Read the model definition and answer for the solid it produces. Units are mm, in the model's axes. Face numbers are marked on the shaded views. A direction names the side the tool comes from. Round coordinates to 2 decimals unless told otherwise and drop trailing zeros. Write each loop counter-clockwise with the first axis right and the second up, starting at its lowest first coordinate (ties: lowest second). Pieces come first, ordered by that corner, then holes. Notation, with made-up numbers: (-1.75, 47.25) -> (9.25, 47.25) arc R18 cw to (9.25, 72.25) -> close; hole circle Ø3 at (55, 40.5). An arc over 180 degrees is marked (long way). Return JSON: item names as keys, results as strings.
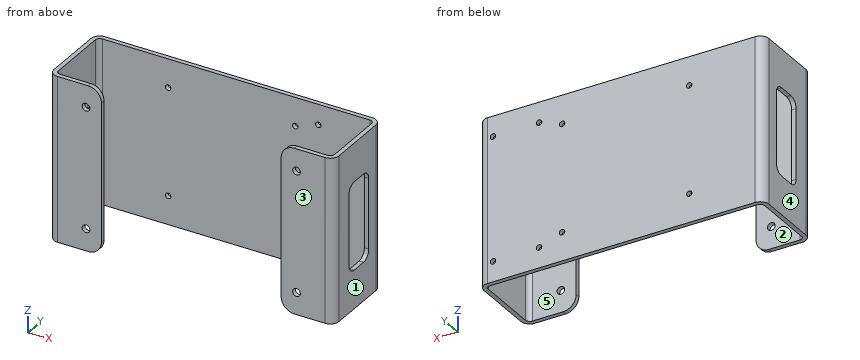
from build123d import *

# Parameters (mm, degrees)
SKETCH1_W                    = 130
SKETCH1_H                    = 75
BASE_FLANGE1_DEPTH           = 2
EDGE_FLANGE1_STRIP_W         = 12
EDGE_FLANGE1_STRIP_H         = 2
EDGE_FLANGE1_STRIP_CUT_DEPTH = 75
EDGE_FLANGE1_DEPTH           = 75
EDGE_FLANGE2_STRIP_W         = 12
EDGE_FLANGE2_STRIP_H         = 2
EDGE_FLANGE2_STRIP_CUT_DEPTH = 75
EDGE_FLANGE2_DEPTH           = 75
EDGE_FLANGE3_STRIP_W         = 12
EDGE_FLANGE3_STRIP_H         = 2
EDGE_FLANGE3_STRIP_CUT_DEPTH = 75
EDGE_FLANGE3_DEPTH           = 75
EDGE_FLANGE4_STRIP_W         = 12
EDGE_FLANGE4_STRIP_H         = 2
EDGE_FLANGE4_STRIP_CUT_DEPTH = 75
EDGE_FLANGE4_DEPTH           = 75
SKETCH20_R                   = 1.75
CUT_EXTRUDE1_DEPTH           = 2
CUT_EXTRUDE2_DEPTH           = 128
FILLET1_R                    = 6
SKETCH22_R                   = 1.25
CUT_EXTRUDE3_DEPTH           = 2
SKETCH23_R                   = 1.25
CUT_EXTRUDE4_DEPTH           = 2


# Sheet-metal steps are written as plain solids
with BuildPart() as part:
    # Sketch1 → Base-Flange1 (new body)
    with BuildSketch(Plane(origin=(0, 0, 0), x_dir=(1, 0, 0), z_dir=(0, 1, 0))):
        Rectangle(SKETCH1_W, SKETCH1_H)
    extrude(amount=-BASE_FLANGE1_DEPTH)

    # Edge-Flange1 strip (across the edge) → Edge-Flange1 strip cut (cut)
    with BuildSketch(Plane(origin=(-65, -2, 37.5), x_dir=(1, 0, 0), z_dir=(0, 0, -1))):
        with Locations((-2, -1)):
            Rectangle(EDGE_FLANGE1_STRIP_W, EDGE_FLANGE1_STRIP_H)
    extrude(amount=EDGE_FLANGE1_STRIP_CUT_DEPTH, mode=Mode.SUBTRACT)

    # Edge-Flange1 section (across the edge) → Edge-Flange1 (add)
    with BuildSketch(Plane(origin=(-65, -2, 37.5), x_dir=(1, 0, 0), z_dir=(0, 0, -1))):
        with BuildLine():
            Line((0, 2), (0, 32))
            Line((0, 32), (2, 32))
            Line((2, 32), (2, 2))
            ThreePointArc((2, 2), (2.585786438, 0.585786438), (4, 0))
            Line((4, 0), (4, -2))
            ThreePointArc((4, -2), (1.171572875, -0.828427125), (0, 2))
        make_face()
    extrude(amount=EDGE_FLANGE1_DEPTH)

    # Edge-Flange2 strip (across the edge) → Edge-Flange2 strip cut (cut)
    with BuildSketch(Plane(origin=(-63, -34, 37.5), x_dir=(0, 1, 0), z_dir=(0, 0, -1))):
        with Locations((-4, -1)):
            Rectangle(EDGE_FLANGE2_STRIP_W, EDGE_FLANGE2_STRIP_H)
    extrude(amount=EDGE_FLANGE2_STRIP_CUT_DEPTH, mode=Mode.SUBTRACT)

    # Edge-Flange2 section (across the edge) → Edge-Flange2 (add)
    with BuildSketch(Plane(origin=(-63, -34, 37.5), x_dir=(0, 1, 0), z_dir=(0, 0, -1))):
        with BuildLine():
            Line((-2, 2), (-2, 22))
            Line((-2, 22), (0, 22))
            Line((0, 22), (0, 2))
            ThreePointArc((0, 2), (0.585786438, 0.585786438), (2, 0))
            Line((2, 0), (2, -2))
            ThreePointArc((2, -2), (-0.828427125, -0.828427125), (-2, 2))
        make_face()
    extrude(amount=EDGE_FLANGE2_DEPTH)

    # Edge-Flange3 strip (across the edge) → Edge-Flange3 strip cut (cut)
    with BuildSketch(Plane(origin=(65, -2, -37.5), x_dir=(-1, 0, 0), z_dir=(0, 0, 1))):
        with Locations((-2, -1)):
            Rectangle(EDGE_FLANGE3_STRIP_W, EDGE_FLANGE3_STRIP_H)
    extrude(amount=EDGE_FLANGE3_STRIP_CUT_DEPTH, mode=Mode.SUBTRACT)

    # Edge-Flange3 section (across the edge) → Edge-Flange3 (add)
    with BuildSketch(Plane(origin=(65, -2, -37.5), x_dir=(-1, 0, 0), z_dir=(0, 0, 1))):
        with BuildLine():
            Line((0, 2), (0, 32))
            Line((0, 32), (2, 32))
            Line((2, 32), (2, 2))
            ThreePointArc((2, 2), (2.585786438, 0.585786438), (4, 0))
            Line((4, 0), (4, -2))
            ThreePointArc((4, -2), (1.171572875, -0.828427125), (0, 2))
        make_face()
    extrude(amount=EDGE_FLANGE3_DEPTH)

    # Edge-Flange4 strip (across the edge) → Edge-Flange4 strip cut (cut)
    with BuildSketch(Plane(origin=(63, -34, -37.5), x_dir=(0, 1, 0), z_dir=(0, 0, 1))):
        with Locations((-4, -1)):
            Rectangle(EDGE_FLANGE4_STRIP_W, EDGE_FLANGE4_STRIP_H)
    extrude(amount=EDGE_FLANGE4_STRIP_CUT_DEPTH, mode=Mode.SUBTRACT)

    # Edge-Flange4 section (across the edge) → Edge-Flange4 (add)
    with BuildSketch(Plane(origin=(63, -34, -37.5), x_dir=(0, 1, 0), z_dir=(0, 0, 1))):
        with BuildLine():
            Line((-2, 2), (-2, 22))
            Line((-2, 22), (0, 22))
            Line((0, 22), (0, 2))
            ThreePointArc((0, 2), (0.585786438, 0.585786438), (2, 0))
            Line((2, 0), (2, -2))
            ThreePointArc((2, -2), (-0.828427125, -0.828427125), (-2, 2))
        make_face()
    extrude(amount=EDGE_FLANGE4_DEPTH)

    # Sketch20 → Cut-Extrude1 (cut)
    with BuildSketch(Plane(origin=(0, -34, 0), x_dir=(1, 0, 0), z_dir=(0, 1, 0))):
        with Locations(Location((-48, -27.5, 0), (0, 0, 180))):
            Circle(SKETCH20_R)
        with Locations(Location((-48, 27.5, 0), (0, 0, 180))):
            Circle(SKETCH20_R)
    cut_extrude1 = extrude(amount=-CUT_EXTRUDE1_DEPTH, mode=Mode.SUBTRACT)

    # Sketch21 → Cut-Extrude2 (cut)
    with BuildSketch(Plane.ZY.offset(65)):
        with BuildLine():
            Line((-16, -9.5), (16, -9.5))
            ThreePointArc((16, -9.5), (18.828427125, -10.671572875), (20, -13.5))
            Line((20, -13.5), (20, -20.5))
            ThreePointArc((20, -20.5), (18.828427125, -23.328427125), (16, -24.5))
            Line((16, -24.5), (-16, -24.5))
            ThreePointArc((-16, -24.5), (-18.828427125, -23.328427125), (-20, -20.5))
            Line((-20, -20.5), (-20, -13.5))
            ThreePointArc((-20, -13.5), (-18.828427125, -10.671572875), (-16, -9.5))
        make_face()
    cut_extrude2 = extrude(amount=-CUT_EXTRUDE2_DEPTH, mode=Mode.SUBTRACT)

    # Fillet1
    fillet1_edges = [part.edges().sort_by_distance(p)[0] for p in [
        (41, -35, -37.5),
        (41, -35, 37.5),
        (-41, -35, 37.5),
        (-41, -35, -37.5),
    ]]
    fillet(fillet1_edges, radius=FILLET1_R)

    # Mirror4: Cut-Extrude1, Cut-Extrude2 across plane
    add(cut_extrude1.mirror(Plane(origin=(0, 0, 0), x_dir=(0, 0, 1), z_dir=(1, 0, 0))), mode=Mode.SUBTRACT)
    add(cut_extrude2.mirror(Plane(origin=(0, 0, 0), x_dir=(0, 0, 1), z_dir=(1, 0, 0))), mode=Mode.SUBTRACT)

    # Sketch22 → Cut-Extrude3 (cut)
    with BuildSketch(Plane(origin=(0, 0, 0), x_dir=(1, 0, 0), z_dir=(0, 1, 0))):
        with BuildLine():
            Line((-31, 23.25), (-31, 24.5))
            Line((-31, 24.5), (-29.75, 24.5))
            ThreePointArc((-29.75, 24.5), (-31.883883476, 25.383883476), (-31, 23.25))
        make_face()
        with BuildLine():
            Line((-29.75, 24.5), (-31, 24.5))
            Line((-31, 24.5), (-31, 23.25))
            ThreePointArc((-31, 23.25), (-30.116116524, 23.616116524), (-29.75, 24.5))
        make_face()
        with Locations(Location((27, 24.5, 0), (0, 0, 270))):
            Circle(SKETCH22_R)
        with Locations(Location((27, -24.5, 0), (0, 0, 270))):
            Circle(SKETCH22_R)
        with Locations(Location((-31, -24.5, 0), (0, 0, 270))):
            Circle(SKETCH22_R)
    extrude(amount=-CUT_EXTRUDE3_DEPTH, mode=Mode.SUBTRACT)

    # Sketch23 → Cut-Extrude4 (cut)
    with BuildSketch(Plane(origin=(0, 0, 0), x_dir=(1, 0, 0), z_dir=(0, 1, 0))):
        with BuildLine():
            ThreePointArc((38.75, -28.25), (38.383883476, -27.366116524), (37.5, -27))
            Line((37.5, -27), (37.5, -28.25))
            Line((37.5, -28.25), (38.75, -28.25))
        make_face()
        with BuildLine():
            Line((37.5, -28.25), (37.5, -27))
            ThreePointArc((37.5, -27), (36.616116524, -29.133883476), (38.75, -28.25))
            Line((38.75, -28.25), (37.5, -28.25))
        make_face()
        with Locations(Location((37.5, 28.25, 0), (0, 0, 270))):
            Circle(SKETCH23_R)
        with Locations(Location((58.5, 28.25, 0), (0, 0, 270))):
            Circle(SKETCH23_R)
        with Locations(Location((58.5, -28.25, 0), (0, 0, 270))):
            Circle(SKETCH23_R)
    extrude(amount=-CUT_EXTRUDE4_DEPTH, mode=Mode.SUBTRACT)


solid = part.part
Item 1: Section A-A (z = -4) is taken. Give the vertices of the cut face in (x, y).
Worked answers:
{"outline": "(-65, -32) arc R4 ccw to (-61, -36) -> (-41, -36) -> (-41, -34) -> (-61, -34) arc R2 cw to (-63, -32) -> (-63, -24.5) -> (-65, -24.5) -> close; (-65, -9.5) -> (-63, -9.5) -> (-63, -4) arc R2 cw to (-61, -2) -> (61, -2) arc R2 cw to (63, -4) -> (63, -9.5) -> (65, -9.5) -> (65, -4) arc R4 ccw to (61, 0) -> (-61, 0) arc R4 ccw to (-65, -4) -> close; (41, -36) -> (61, -36) arc R4 ccw to (65, -32) -> (65, -24.5) -> (63, -24.5) -> (63, -32) arc R2 cw to (61, -34) -> (41, -34) -> close"}
Item 2: Section D-D (y = -29.5) is taken. Give the vertices of the cut face in (x, z), then the cut area to 3 significant figures.
Worked answers:
{"outline": "(-65, -37.5) -> (-63, -37.5) -> (-63, 37.5) -> (-65, 37.5) -> close; (63, -37.5) -> (65, -37.5) -> (65, 37.5) -> (63, 37.5) -> close", "area": "300 mm2"}
Item 3: Straight lines are drawn through the part: L1, parallel to Z at x = -48, y = -35.05; L2, parallel to Y at x = 48, z = -14.5; L3, parallel to X at y = -8, z = -23.5. For each, find the intervals that lie inside material, in ascending order. Write a range as [from, to].
Worked answers:
{"L1": "z = [-37.5, -29.25], [-25.75, 25.75], [29.25, 37.5]", "L2": "y = [-36, -34], [-2, 0]", "L3": "x = [-65, -63], [63, 65]"}
Item 4: Section C-C (x = 58.5) is taken. Give the vertices of the cut face in (y, z).
Worked answers:
{"outline": "(-36, -37.5) -> (-34, -37.5) -> (-34, 37.5) -> (-36, 37.5) -> close; (-2, -37.5) -> (0, -37.5) -> (0, -29.5) -> (-2, -29.5) -> close; (-2, -27) -> (0, -27) -> (0, 27) -> (-2, 27) -> close; (-2, 29.5) -> (0, 29.5) -> (0, 37.5) -> (-2, 37.5) -> close"}
Item 5: A tool of negligible diameter and unlimited length cuts with its end or side. For the marked faces 4 and 5, from which of +Z, -Z, +X, -X, +Y, -Y can it reach the whole face along a straight path? Write none if from no direction.
Worked answers:
{"face 4": "+Z, -Z, -X, +Y, -Y", "face 5": "+Z, -Z"}
Item 6: Flat-ended cylindrical pins translate along their axes: pin 1 (3 mm diameter, centred on x = 17.5, z = 28, fed in from -Y); pin 2 (2 mm diameter, centred on x = 63.5, z = -6, fed in from -Y); pin 3 (8 mm diameter, centred on x = 38, z = 12, fed in from +Y); pin 4 (1.6 mm diameter, centred on y = -35, z = -15, fed in from +X). Find the tip coordinate at first contact, or state that the pin passes through.
Worked answers:
{"pin 1": "stops at y = -2", "pin 2": "stops at y = -35.71", "pin 3": "stops at y = 0", "pin 4": "stops at x = 64.34"}
Item 7: Section B-B (y = -18) is taken. Give the vertices of the cut face in (x, z).
Worked answers:
{"outline": "(-65, -37.5) -> (-63, -37.5) -> (-63, -20) -> (-65, -20) -> close; (-65, 20) -> (-63, 20) -> (-63, 37.5) -> (-65, 37.5) -> close; (63, -37.5) -> (65, -37.5) -> (65, -20) -> (63, -20) -> close; (63, 20) -> (65, 20) -> (65, 37.5) -> (63, 37.5) -> close"}
Item 8: For a pull along Y with two mould halves and no side action, classify the marked faces 1, 2 and 3 as released by +Y, released by -Y, zero draft, split by the parting line, or undercut.
Worked answers:
{"face 1": "zero draft", "face 2": "undercut", "face 3": "released by -Y"}
